The listing builds one solid part. Answer for the finished solid, in the listing's coordinates (mm). Round coordinates to 2 decimals unless told otherwise and drop trailing zeros. Order: outer loops, then holes, each group sorted by start corner. A loop starts at its lowest first (then second) coordinate and runs counter-clockwise, first axis right, second up. Notation, with made-up numbers: (56, -6) - (97, -6) arc R28 cw to (97, 26) - close; hole circle Ø7 at (14, 3.25). An arc over 180 degrees is marked (long way). Write item = value, one per line.
Autodesk Inventor part; units mm, degrees
ref_plane "YZ Plane" through (0, 0, 0) normal (1, 0, 0) x (0, 1, 0)
ref_plane "XZ Plane" through (0, 0, 0) normal (0, 1, 0) x (-1, 0, 0)
ref_plane "XY Plane" through (0, 0, 0) normal (0, 0, 1) x (1, 0, 0)
sketch "Sketch1" plane through (0, 0, 0) normal (0, 1, 0) x (-1, 0, 0)
  circle A0 centre (0, 0) radius 65
  circle A1 centre (0, 0) radius 85
  line L0 (0, 0) -> (28.7013, -69.291)
  line L1 (0, 0) -> (0, -65)
  circle A2 centre (28.7013, -69.291) radius 3.5
  circle A3 centre (69.291, -28.7013) radius 3.5
  circle A4 centre (69.291, 28.7013) radius 3.5
  circle A5 centre (28.7013, 69.291) radius 3.5
  circle A6 centre (-28.7013, 69.291) radius 3.5
  circle A7 centre (-69.291, 28.7013) radius 3.5
  circle A8 centre (-69.291, -28.7013) radius 3.5
  circle A9 centre (-28.7013, -69.291) radius 3.5
  dimension "d0" = 130
  dimension "d1" = 170
  dimension "d2" = 22.5
  dimension "d3" = 75
  dimension "d4" = 7
  dimension "d7" = 360
extrude "Extrusion1" add sketch "Sketch1" along normal blind 1
equation "\"d3\" = 0.25 * d0 + 0.25 * d1"
properties part number "Velcro connection"
Q1. A flat-ended cylindrical pin translates along its axis: P1, Ø5.5, axis at x = 28.7, z = -69.29, coming from the +Y side. Find the tip coordinate at first contact, or state that the pin passes through.
Model answer:
P1 = through
Q2. Determine the mould class of faces 1 (the face through (67.453, 0.493, 51.721)), 2 (the face through (19, 1, -63)), 3 (the face through (66.06, 0.49, -27.36)) for opening direction Z: released by +Z, released by -Z, zero draft, split by the parting line, or undercut.
Model answer:
face_1 = split by the parting line
face_2 = zero draft
face_3 = undercut
Q3. Section A-A on x = 0 is taken. Determine the outline of the cut face in (y, z).
Model answer:
outline = (0, -85) - (1, -85) - (1, -65) - (0, -65) - close; (0, 65) - (1, 65) - (1, 85) - (0, 85) - close
Q4. Section B-B on z = 0 is taken. Determine the outline of the cut face in (x, y), then the cut area to 3 significant figures.
Model answer:
outline = (-85, 0) - (-65, 0) - (-65, 1) - (-85, 1) - close; (65, 0) - (85, 0) - (85, 1) - (65, 1) - close
area = 40.0 mm^2
Q5. Section C-C on y = 0.85 is taken. Count the separate pieces of the cut face and the enclosed holes in it, then the cut area to 3 significant figures.
Model answer:
separate_pieces = 1
enclosed_holes = 9
area = 9,120 mm^2
Q6. Find the intervals of material crossed by line 1 (Z direction, x = 0, y = 0.6); line 2 (Z direction, x = 31.5, y = 0.1); line 3 (X direction, y = 0.6, z = 16.5), in increasing order. Write a range as from..to.
Model answer:
line_1 = -85..-65, 65..85
line_2 = -78.95..-71.39, -67.19..-56.86, 56.86..67.19, 71.39..78.95
line_3 = -83.38..-62.87, 62.87..83.38
